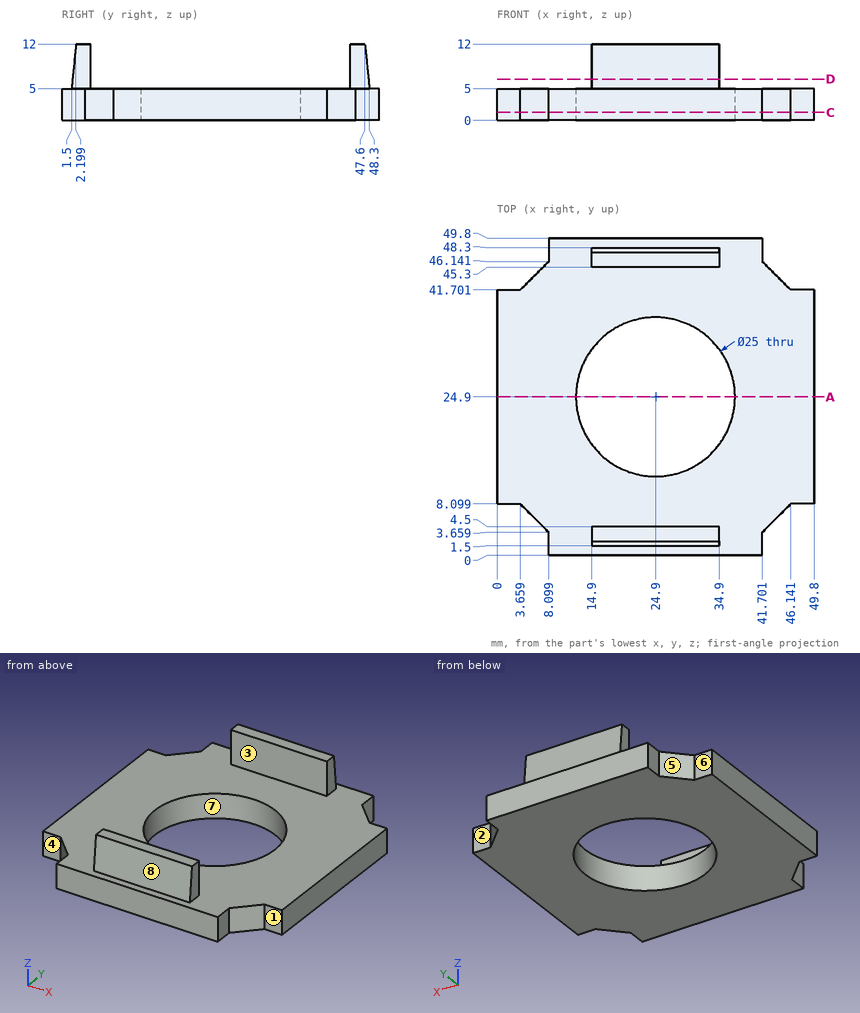
Here's the drawing with two shaded views (mm, measured from the low corner). I have some questions. A direction names the side the tool comes from. Round coordinates to 2 decimals unless told otherwise and drop trailing zeros. Order: outer loops, then holes, each group sorted by start corner. A loop starts at its lowest first (then second) coordinate and runs counter-clockwise, first axis right, second up. Notation, with made-up numbers: (79.5, 38.5) -> (111.5, 38.5) arc R7 ccw to (111.5, 46.5) -> close; hole circle Ø1 at (-20, 7). An arc over 180 degrees is marked (long way). Write each question's results on one line, items separated by ' | '. Start each with the question number.
Item 1: If we section it at D-D, the plane z = 6.5: Write out the boundary of the cut face in (x, y).
Item 2: If we section it at A-A, the plane y = 24.9: Write out the boundary of the cut face in (x, z), then the cut area to 3 significant figures.
Item 3: Please list where these lines run through material, in increasing order: L1, parallel to Y at x = 24.9, z = 2.4; L2, parallel to Z at x = 40.5, y = 23.
Item 4: If we section it at C-C, the plane z = 1.25: Write out the boundary of the cut face in (x, y), then the cut area to 3 significant figures.
Item 5: Which directions (+Z, -Z, +X, -X, +Y, -Y) give clear straight access to the entire face, cutting with the end or side of a thin tool? Please do the marked faces 1, 2, 3, 4 and 5.
Item 6: Thinking about a two-plate mould opening in Y: for the marked faces 6, 7 and 8, which applies, +Y half, -Y half, draft (parallel to the pull), parting line (faces both ways), or undercut?
Item 7: Will these pins go through, and if not, where does the flat tip stop? pin 1 (4 mm diameter, centred on x = 11.5, y = 12.5, fed in from -Z); pin 2 (3 mm diameter, centred on y = 48, z = 2.5, fed in from -X); pin 3 (4 mm diameter, centred on x = 48.5, z = 1.5, fed in from +Y); pin 4 (0.9 mm diameter, centred on y = 3.5, z = 8.5, fed in from +X).
Results:
1) outline: (14.9, 1.65) -> (34.9, 1.65) -> (34.9, 4.5) -> (14.9, 4.5) -> close; (14.9, 45.3) -> (34.9, 45.3) -> (34.9, 48.15) -> (14.9, 48.15) -> close
2) outline: (0, 0) -> (12.4, 0) -> (12.4, 5) -> (0, 5) -> close; (37.4, 0) -> (49.8, 0) -> (49.8, 5) -> (37.4, 5) -> close | area: 124 mm2
3) L1: y = 0 to 12.4, 37.4 to 49.8 | L2: z = 0 to 5
4) outline: (0, 8.1) -> (3.66, 8.1) -> (8.1, 3.66) -> (8.1, 0) -> (41.7, 0) -> (41.7, 3.66) -> (46.14, 8.1) -> (49.8, 8.1) -> (49.8, 41.7) -> (46.14, 41.7) -> (41.7, 46.14) -> (41.7, 49.8) -> (8.1, 49.8) -> (8.1, 46.14) -> (3.66, 41.7) -> (0, 41.7) -> close; hole circle Ø25 at (24.9, 24.9) | area: 1,770 mm2
5) face 1: +Z, -Z, +X, -Y | face 2: +Z, -Z, +X, +Y | face 3: +Z, +X, -X | face 4: +Z, -Z, -X, -Y | face 5: +Z, -Z, -X, +Y
6) face 6: +Y half | face 7: undercut | face 8: -Y half
7) pin 1: stops at z = 0 | pin 2: stops at x = 8.1 | pin 3: stops at y = 41.7 | pin 4: stops at x = 34.9
